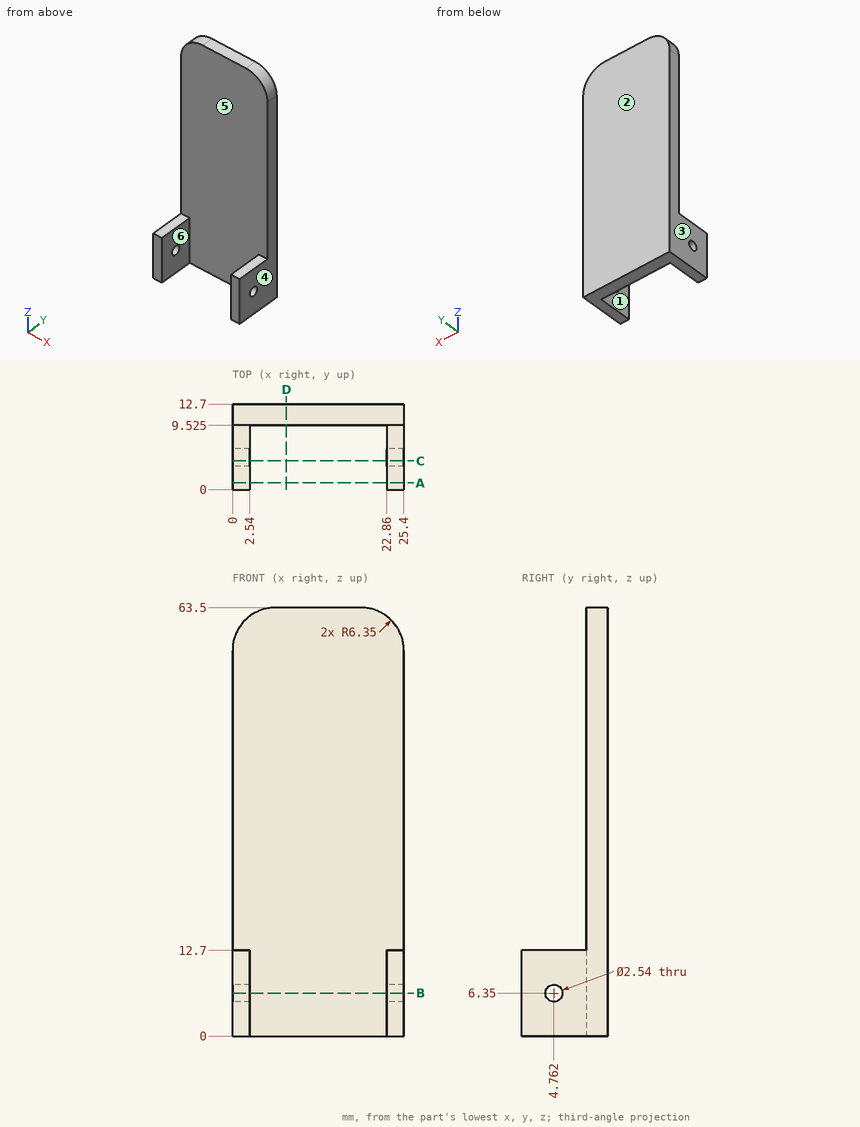
Source: three-view drawing plus pictorial views. Frame: mm from the lowest corner of the part. A direction names the side the tool comes from. Coordinates: 2 decimals unless noted, no trailing zeros. Loops run counter-clockwise (first coordinate to the right, second up) from the corner with the lowest first, then second, coordinate; pieces in that order, holes last. Notation, with made-up numbers: (-28.5, 85) - (-11.5, 85) arc R29 cw to (-11.5, 122) - close; hole circle Ø5 at (18.5, -26). An arc over 180 degrees is marked (long way). One line per item, written item: value. Start each with the question number.
1. Contact query for flat-ended pins moving along their axis: P1, Ø12, axis at x = 11.5, z = 11, coming from the -Y side (1 decimal); P2, Ø3, axis at x = 1.5, y = 3, coming from the +Z side. Output: stop coordinate, or through.
2. Section C-C (y = 4.25). Return the cut outline in (x, z).
3. Section A-A (y = 1). Return the cut outline in (x, z).
4. Section D-D (x = 8). Return the cut outline in (y, z) (1 decimal).
5. Ray query, L1, parallel to X at y = 6, z = 11; L2, parallel to Z at x = 2.5, y = 4.75; L3, parallel to Y at x = 3, z = 32 (1 decimal). Return the intervals inside material, ascending.
6. Section B-B (z = 6.35). Return the cut outline in (x, y) (1 decimal).
7. Set-up query: the marked faces 1 and 2. Return all of +Z, -Z, +X, -X, +Y, -Y with unobstructed straight access to the full face (end or side cutting, diameter ignored); none if empty.
8. Mould query, pull axis X, two halves, no side actions, for the marked faces 3, 4, 5 and 6. Classes: pulls with the +X half, pulls with the -X half, needs draft (parallel to the pull), parting line crosses it, or undercut.
Verdict:
1. P1: stops at y = 9.5
1. P2: stops at z = 12.7
2. outline: (0, 0) - (2.54, 0) - (2.54, 5.19) - (0, 5.19) - close; (0, 7.51) - (2.54, 7.51) - (2.54, 12.7) - (0, 12.7) - close; (22.86, 0) - (25.4, 0) - (25.4, 5.19) - (22.86, 5.19) - close; (22.86, 7.51) - (25.4, 7.51) - (25.4, 12.7) - (22.86, 12.7) - close
3. outline: (0, 0) - (2.54, 0) - (2.54, 12.7) - (0, 12.7) - close; (22.86, 0) - (25.4, 0) - (25.4, 12.7) - (22.86, 12.7) - close
4. outline: (9.5, 0) - (12.7, 0) - (12.7, 63.5) - (9.5, 63.5) - close
5. L1: x = 0 to 2.54, 22.86 to 25.4
5. L2: z = 0 to 5.08, 7.62 to 12.7
5. L3: y = 9.5 to 12.7
6. outline: (0, 0) - (2.5, 0) - (2.5, 3.5) - (0, 3.5) - close; (0, 6) - (2.5, 6) - (2.5, 9.5) - (22.9, 9.5) - (22.9, 6) - (25.4, 6) - (25.4, 12.7) - (0, 12.7) - close; (22.9, 0) - (25.4, 0) - (25.4, 3.5) - (22.9, 3.5) - close
7. face 1: +Z, -Z, -Y
7. face 2: +Z, -Z, +X, -X, +Y
8. face 3: pulls with the -X half
8. face 4: pulls with the +X half
8. face 5: undercut
8. face 6: undercut
